Could you check a few things on this drawing? It's one solid part, dimensions in mm from its lowest x, y, z. A direction names the side the tool comes from. Round coordinates to 2 decimals unless told otherwise and drop trailing zeros. Order: outer loops, then holes, each group sorted by start corner. A loop starts at its lowest first (then second) coordinate and runs counter-clockwise, first axis right, second up.
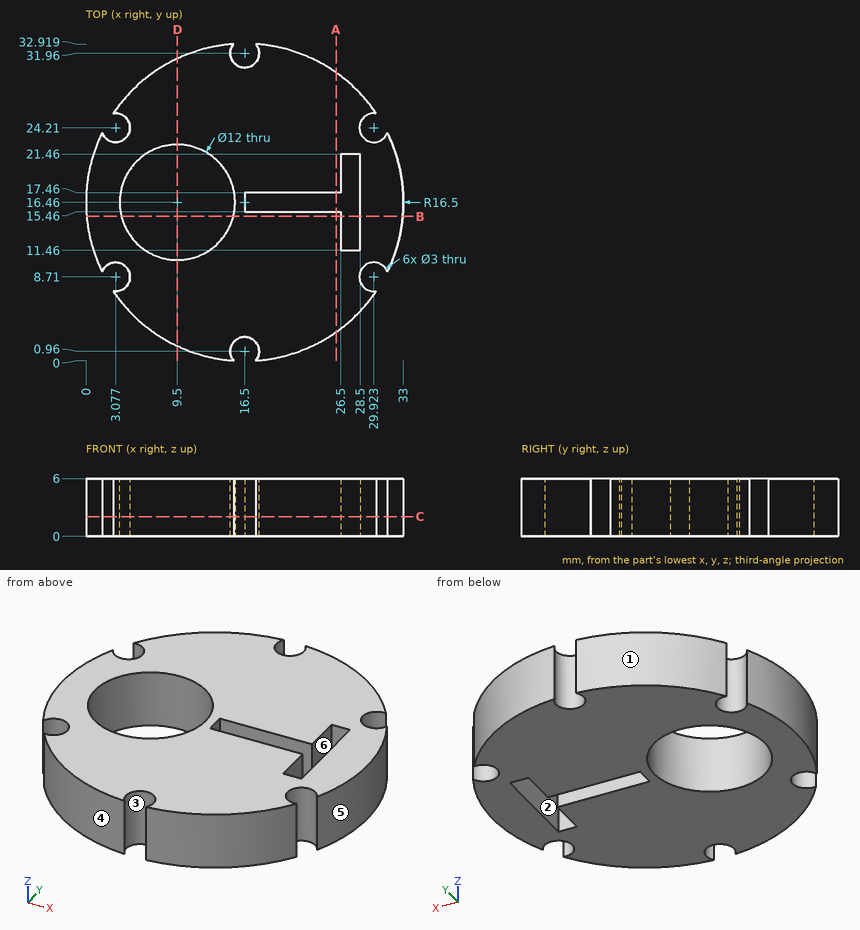
(1) I want a section at B-B, the plane y = 15. List the corners of the cut face in (x, z) for me (1 decimal), plus the area to 3 significant figures.
(2) Please list where these lines run through material, in increasing order: probe 1 along X at (y, z) = (11.5, 1.45) (1 decimal); probe 2 along X at (y, z) = (10, 4) (1 decimal); probe 3 along Y at (x, z) = (3, 5.65) (1 decimal).
(3) I want a section at C-C, the plane z = 2.05. List the corners of the cut face in (x, y) for me.
(4) I want a section at D-D, the plane x = 9.5. List the corners of the cut face in (y, z) for me, plus the area to 3 significant figures.
(5) On a 3-axis mill with a long thin cutter (end or side, diameter ignored), from which of +Z, -Z, +X, -X, +Y, -Y can I reach the whole of each face in a straight line? I mean the marked faces 5 and 6. Say none if no direction works.
(6) I'm going to push flat-ended pins straight in: pin 1 Ø1.8 at (y, z) = (15, 4.5) entering from -X; pin 2 Ø2 at (y, z) = (19.5, 3) entering from +X; pin 3 Ø2 at (x, z) = (10.5, 2.5) entering from +Y. Where does each tip first touch, or does it pass through?
(7) If we mould it in two halves opening along Y, with no side actions, what happens to the marked faces 1, 2, 3 and 4? For each: pulls with the +Y half, pulls with the -Y half, needs draft (parallel to the pull), parting line crosses it, or undercut.
(8) I want a section at A-A, the plane x = 26. List the corners of the cut face in (y, z) for me, plus the area to 3 significant figures.
Ans:
1. outline: (0.1, 0) - (3.7, 0) - (3.7, 6) - (0.1, 6) - close; (15.3, 0) - (26.5, 0) - (26.5, 6) - (15.3, 6) - close; (28.5, 0) - (32.9, 0) - (32.9, 6) - (28.5, 6) - close
1. area: 115 mm2
2. probe 1: x = 0.8 to 6.1, 12.9 to 26.5, 28.5 to 32.2
2. probe 2: x = 1.3 to 2.3, 3.8 to 29.2, 30.7 to 31.7
2. probe 3: y = 7 to 7.2, 10.2 to 22.7, 25.7 to 25.9
3. outline: (1.67, 9.23) arc R1.5 cw (long way) to (2.82, 7.23) arc R16.5 ccw to (15.35, 0) arc R1.5 cw (long way) to (17.65, 0) arc R16.5 ccw to (30.18, 7.23) arc R1.5 cw (long way) to (31.33, 9.23) arc R16.5 ccw to (31.33, 23.69) arc R1.5 cw (long way) to (30.18, 25.69) arc R16.5 ccw to (17.65, 32.92) arc R1.5 cw (long way) to (15.35, 32.92) arc R16.5 ccw to (2.82, 25.69) arc R1.5 cw (long way) to (1.67, 23.69) arc R16.5 ccw to start; hole circle Ø12 at (9.5, 16.46); hole (16.5, 15.46) - (26.5, 15.46) - (26.5, 11.46) - (28.5, 11.46) - (28.5, 21.46) - (26.5, 21.46) - (26.5, 17.46) - (16.5, 17.46) - close
4. outline: (1.52, 0) - (10.46, 0) - (10.46, 6) - (1.52, 6) - close; (22.46, 0) - (31.4, 0) - (31.4, 6) - (22.46, 6) - close
4. area: 107 mm2
5. face 5: +Z, -Z, +X
5. face 6: +Z, -Z
6. pin 1: stops at x = 0.01
6. pin 2: stops at x = 32.87
6. pin 3: stops at y = 32.18
7. face 1: pulls with the +Y half
7. face 2: undercut
7. face 3: undercut
7. face 4: pulls with the -Y half
8. outline: (2.97, 0) - (15.46, 0) - (15.46, 6) - (2.97, 6) - close; (17.46, 0) - (29.95, 0) - (29.95, 6) - (17.46, 6) - close
8. area: 150 mm2
